```python
from build123d import *

# Parameters (mm, degrees)
CORTAR_EXTRUIR1_DEPTH      = 77.200073819
CORTAR_EXTRUIR1_DEPTH_BACK = 77.200073819
CROQUIS2_R                 = 2.25
REDONDEO1_R                = 0.3
CHAFL_N1_SIZE              = 1
CHAFL_N1_SIZE2             = 1.732050808
REDONDEO2_R                = 0.3


with BuildPart() as part:
    # Croquis1 → Revolución1 (revolve)
    with BuildSketch(Plane(origin=(0, 0, 0), x_dir=(0, 0, -1), z_dir=(1, 0, 0)), mode=Mode.PRIVATE) as revoluci_n1_sk:
        Polygon((0, 0), (0, 9.525), (3, 9.525), (3, 8), (75, 8), (75, 0), align=None)
    revolve(revoluci_n1_sk.sketch.rotate(Axis((0, 0, 0), (0, 0, -1)), 90), axis=Axis((0, 0, 0), (0, 0, -1)))

    # Croquis2 → Cortar-Extruir1 (cut, two sides: drawn at the far end of the back side and taken through both)
    with BuildSketch(Plane(origin=(0, 0, 0), x_dir=(1, 0, 0), z_dir=(0, 1, 0)).offset(-CORTAR_EXTRUIR1_DEPTH_BACK)):
        with Locations(Location((0, 68.25, 0), (0, 0, 270))):
            Circle(CROQUIS2_R)
    extrude(amount=CORTAR_EXTRUIR1_DEPTH + CORTAR_EXTRUIR1_DEPTH_BACK, mode=Mode.SUBTRACT)

    # Redondeo1
    redondeo1_edges = [part.edges().sort_by_distance(p)[0] for p in [
        (-8, 0, -3),
    ]]
    fillet(redondeo1_edges, radius=REDONDEO1_R)

    # Chaflán1
    chafl_n1_edges = [part.edges().sort_by_distance(p)[0] for p in [
        (-8, 0, -75),
    ]]
    chafl_n1_side = [part.faces().sort_by_distance(p)[0] for p in [
        (0, 0, -75),
    ]]
    chamfer(chafl_n1_edges, length=CHAFL_N1_SIZE, length2=CHAFL_N1_SIZE2, reference=chafl_n1_side[0])

    # Redondeo2
    redondeo2_edges = [part.edges().sort_by_distance(p)[0] for p in [
        (-9.525, 0, -3),
        (-9.525, 0, 0),
    ]]
    fillet(redondeo2_edges, radius=REDONDEO2_R)


solid = part.part
```
The listing builds one solid part. Answer for the finished solid, in the listing's coordinates (mm). A direction names the side the tool comes from. Give positions to 0.01 mm unless a question says otherwise; leave off trailing zeros. Write each loop counter-clockwise with the first axis right and the second up, starting at its lowest first coordinate (ties: lowest second). Pieces come first, ordered by that corner, then holes. Notation, with made-up numbers: (-37, -8.75) - (-32, -8.75) arc R12 ccw to (-32, -3.75) - close; hole circle Ø5 at (24.25, 84). An arc over 180 degrees is marked (long way). Use one line per item in the form item = value. Start each with the question number.
1) Find section C-C on z = -68.25. Determine the outline of the cut face in (x, y).
2) Consider line 1 along Z through (x, y) = (0, -3); line 2 along X through (y, z) = (3.5, -68.25); line 3 along X through (y, z) = (0.75, -68.25). Determine where each line is inside the solid, lowest interval first. Write a range as from..to.
3) Find section D-D on z = -12.5. Determine the outline of the cut face in (x, y), plus the area to 3 significant figures.
4) Find section B-B on y = 0. Determine the outline of the cut face in (x, z) (3 decimals), plus the area to 3 significant figures.
5) The mould has two halves that part along X. Classify faces 1 (the face through (1.52, -0.11, -69.91)), 2 (the face through (3.69, 7.1, -38.77)), 3 (the face through (0, 0, 0)): pulls with the +X half, pulls with the -X half, needs draft (parallel to the pull), parting line crosses it, or undercut.
6) Flat-ended cylindrical pins translate along their axes: pin 1 Ø1.5 at (x, z) = (-4.5, -32) entering from -Y; pin 2 Ø8 at (y, z) = (4, -59) entering from -X; pin 3 Ø4 at (y, z) = (3.5, -37.5) entering from +X. Find the tip coordinate at first contact, or state that the pin passes through.
7) Find section A-A on x = 0. Determine the outline of the cut face in (y, z) (3 decimals), plus the area to 3 significant figures.
8) A tool of negligible diameter and unlimited length cuts with its end or side. For faces 4 (the face through (-8, -3, -3)), 5 (the face through (-2.06, 9.3, -1.52)), from which of +Z, -Z, +X, -X, +Y, -Y can it reach the whole face along a straight path? Write none if from no direction.
Geometry results:
q1.outline = (-2.25, -7.68) - (-2.25, 7.68) arc R8 ccw to start; (2.25, -7.68) arc R8 ccw to (2.25, 7.68) - close
q2.line_1 = -75..-70.5, -66..0
q2.line_2 = -7.19..-2.25, 2.25..7.19
q2.line_3 = -7.96..-2.25, 2.25..7.96
q3.outline = circle Ø16 at (0, 0)
q3.area = 201 mm2
q4.outline = (-9.525, -2.7) arc R0.3 ccw to (-9.225, -3) - (-8.3, -3) arc R0.3 cw to (-8, -3.3) - (-8, -73.268) - (-7, -75) - (7, -75) - (8, -73.268) - (8, -3.3) arc R0.3 cw to (8.3, -3) - (9.225, -3) arc R0.3 ccw to (9.525, -2.7) - (9.525, -0.3) arc R0.3 ccw to (9.225, 0) - (-9.225, 0) arc R0.3 ccw to (-9.525, -0.3) - close; hole circle Ø4.5 at (0, -68.25)
q4.area = 1,190 mm2
q5.face_1 = undercut
q5.face_2 = parting line crosses it
q5.face_3 = needs draft
q6.pin_1 = -7.07
q6.pin_2 = -8
q6.pin_3 = 7.86
q7.outline = (-9.525, -2.7) arc R0.3 ccw to (-9.225, -3) - (-8.3, -3) arc R0.3 cw to (-8, -3.3) - (-8, -66) - (8, -66) - (8, -3.3) arc R0.3 cw to (8.3, -3) - (9.225, -3) arc R0.3 ccw to (9.525, -2.7) - (9.525, -0.3) arc R0.3 ccw to (9.225, 0) - (-9.225, 0) arc R0.3 ccw to (-9.525, -0.3) - close; (-8, -73.268) - (-7, -75) - (7, -75) - (8, -73.268) - (8, -70.5) - (-8, -70.5) - close
q7.area = 1,140 mm2
q8.face_4 = -Z
q8.face_5 = +Z, -Z
